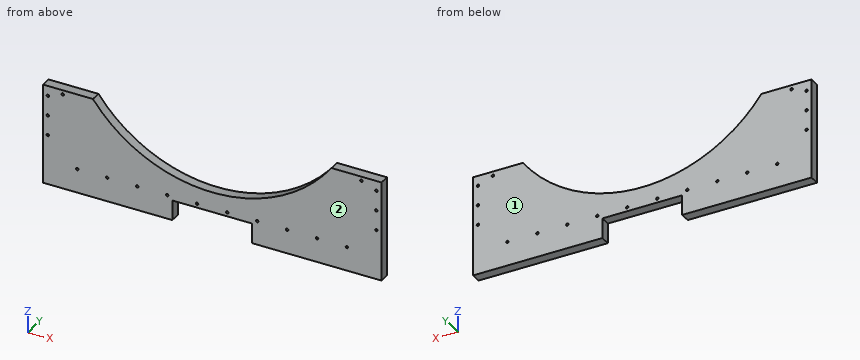
from build123d import *

# Parameters (mm, degrees)
F1_DEPTH = 12.7
F3_D     = 3.175


with BuildPart() as f1:
    # F0 (on Front) → F1 (new body)
    with BuildSketch(Plane.XZ):
        with BuildLine():
            Line((-131.002396, -21.796399), (-194.502396, -21.796399))
            Line((-194.502396, -21.796399), (-194.502396, -148.796399))
            Line((-194.502396, -148.796399), (-30.038724, -148.796399))
            Line((-30.038724, -148.796399), (-30.038724, -123.396399))
            Line((-30.038724, -123.396399), (71.561276, -123.396399))
            Line((71.561276, -123.396399), (71.561276, -148.796399))
            Line((71.561276, -148.796399), (236.024947, -148.796399))
            Line((236.024947, -148.796399), (236.024947, -21.796399))
            Line((236.024947, -21.796399), (172.524947, -21.796399))
            ThreePointArc((172.524947, -21.796399), (20.761276, -97.996399), (-131.002396, -21.796399))
        make_face()
    extrude(amount=F1_DEPTH)

    # F3 (through all)
    with Locations(Plane.XZ.offset(12.7)):
        with Locations((229.674947, -34.496399), (229.674947, -59.896399), (229.674947, -85.296399), (192.211276, -118.316399), (154.111276, -118.316399), (116.011276, -118.316399), (77.911276, -118.316399), (39.811276, -118.316399), (210.624947, -27.102793), (1.471006, -118.316399), (-36.628994, -118.316399), (-74.728994, -118.316399), (-112.828994, -118.316399), (-150.928994, -118.316399), (-188.392666, -85.296399), (-188.392666, -59.896399), (-188.392666, -34.496399), (-169.342666, -27.102793)):
            Hole(F3_D / 2)


solid = f1.part
Source: CAD feature listing. Evaluate the final solid. Frame: model axes, mm. Face numbers are marked on the shaded views. Round coordinates to 2 decimals unless told otherwise and drop trailing zeros. Loops run counter-clockwise (first coordinate to the right, second up) from the corner with the lowest first, then second, coordinate; pieces in that order, holes last. Notation, with made-up numbers: (36.5, 11.5) - (53.5, 11.5) arc R32 ccw to (53.5, 38.5) - close; hole circle Ø1 at (-6.5, 45.25). An arc over 180 degrees is marked (long way). Write item = value, one per line. Start each with the question number.
(1) Pull-direction query (Y, two-part tool) for the marked faces 1 and 2; classes: +Y half, -Y half, draft (parallel to the pull), parting line (faces both ways), or undercut.
(2) Section query A-A, the plane z = -135.5. Output: boundary loops of the cut face in (x, y).
(3) Ray query, line 1 along X through (y, z) = (-2, -138); line 2 along X through (y, z) = (-2.5, -60.5); line 3 along X through (y, z) = (-5.25, -80.5). Return the intervals inside material, ascending. Write a range as from..to.
(4) Section query C-C, the plane z = -48. Output: boundary loops of the cut face in (x, y).
(5) Section query B-B, the plane y = -7.5. State how many separate pieces and enclosed holes the cut face has, plus the area to 3 significant figures.
(6) Pin query (flat end, axial travel): pin 1 (4 mm diameter, centred on x = -188.39, z = -34.5, fed in from +Y); pin 2 (2.5 mm diameter, centred on x = 116.01, z = -118.32, fed in from -Y); pin 3 (1 mm diameter, centred on x = 70.5, y = -10.5, fed in from +Z); pin 4 (6.5 mm diameter, centred on x = 28.5, y = -3.5, fed in from -Z). Return the tip coordinate at first contact, or that it passes through.
(7) Section query D-D, the plane x = 51.5. Output: boundary loops of the cut face in (y, z).
Conclusion:
q1.face_1 = +Y half
q1.face_2 = -Y half
q2.outline = (-194.5, -12.7) - (-30.04, -12.7) - (-30.04, 0) - (-194.5, 0) - close; (71.56, -12.7) - (236.02, -12.7) - (236.02, 0) - (71.56, 0) - close
q3.line_1 = -194.5..-30.04, 71.56..236.02
q3.line_2 = -194.5..-189.86, -186.92..-92.31, 133.83..228.21, 231.14..236.02
q3.line_3 = -194.5..-58.71, 100.23..236.02
q4.outline = (-194.5, -12.7) - (-107.39, -12.7) - (-107.39, 0) - (-194.5, 0) - close; (148.91, -12.7) - (236.02, -12.7) - (236.02, 0) - (148.91, 0) - close
q5.separate_pieces = 1
q5.enclosed_holes = 18
q5.area = 35,800 mm2
q6.pin_1 = 0
q6.pin_2 = through
q6.pin_3 = -91.21
q6.pin_4 = -123.4
q7.outline = (-12.7, -123.4) - (0, -123.4) - (0, -95.48) - (-12.7, -95.48) - close
